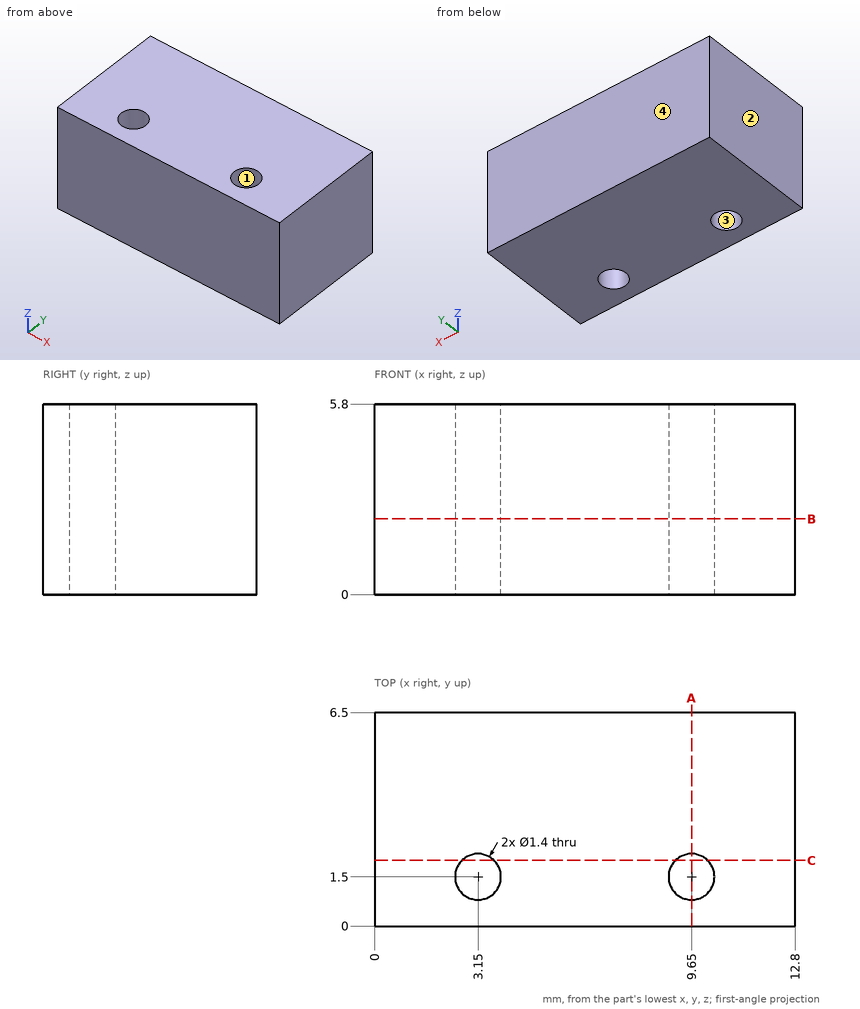
Geometry check sheet. Reference: drawing and pictorial views, mm from the part's lowest x, y, z. Coordinates: 2 decimals unless noted, no trailing zeros. Write each loop counter-clockwise with the first axis right and the second up, starting at its lowest first coordinate (ties: lowest second). Pieces come first, ordered by that corner, then holes. Notation, with made-up numbers: M -23,35.25 L 4,35.25 A29 ccw 4,68.25 Z; hole C 27,78 d8. An arc over 180 degrees is marked long. Write item = value, one per line. Start each with the question number.
1. Thickness scan on probe 1 along Y at (x, z) = (3.15, 2.5); probe 2 along Y at (x, z) = (2.75, 5.3). Record the ranges inside material, lowest first.
2. Mould release check, pull along Y, two halves, no side actions. Record for the marked faces 1, 2, 3 and 4: pulls with the +Y half, pulls with the -Y half, needs draft (parallel to the pull), parting line crosses it, or undercut.
3. Go/stop test with a flat-tipped pin: pin 1 (3 mm diameter, centred on x = 6, y = 5.5, fed in from -Z). Record where the tip stops, or that it passes through.
4. Sectioned sample at C-C (y = 2). Record the cut outline in (x, z), then the cut area to 3 significant figures.
5. Sectioned sample at B-B (z = 2.3). Record the cut outline in (x, y), then the cut area to 3 significant figures.
6. Sectioned sample at A-A (x = 9.65). Record the cut outline in (y, z).
The answers:
q1.probe_1 = 0 to 0.8, 2.2 to 6.5
q1.probe_2 = 0 to 0.93, 2.07 to 6.5
q2.face_1 = undercut
q2.face_2 = needs draft
q2.face_3 = undercut
q2.face_4 = pulls with the +Y half
q3.pin_1 = 0
q4.outline = M 0,0 L 2.66,0 L 2.66,5.8 L 0,5.8 Z; M 3.64,0 L 9.16,0 L 9.16,5.8 L 3.64,5.8 Z; M 10.14,0 L 12.8,0 L 12.8,5.8 L 10.14,5.8 Z
q4.area = 62.9 mm²
q5.outline = M 0,0 L 12.8,0 L 12.8,6.5 L 0,6.5 Z; hole C 3.15,1.5 d1.4; hole C 9.65,1.5 d1.4
q5.area = 80.1 mm²
q6.outline = M 0,0 L 0.8,0 L 0.8,5.8 L 0,5.8 Z; M 2.2,0 L 6.5,0 L 6.5,5.8 L 2.2,5.8 Z
